```python
from build123d import *

# Parameters (mm, degrees)
EXTRUSION1_DEPTH = 18.3
ESQUISSE2_R      = 2
EXTRUSION2_DEPTH = 6.3


with BuildPart() as part:
    # Esquisse1 → Extrusion1 (new body)
    with BuildSketch(Plane.XY):
        with BuildLine():
            Line((0, 0), (30, 0))
            Line((30, 0), (30, 26.1))
            ThreePointArc((30, 26.1), (15, 41.1), (0, 26.1))
            Line((0, 26.1), (0, 0))
        make_face()
    extrude(amount=-EXTRUSION1_DEPTH)

    # Esquisse2 → Extrusion2 (cut)
    with BuildSketch(Plane.XY):
        with Locations((15, 26.6)):
            Circle(ESQUISSE2_R)
    extrude(amount=-EXTRUSION2_DEPTH, mode=Mode.SUBTRACT)


solid = part.part
```
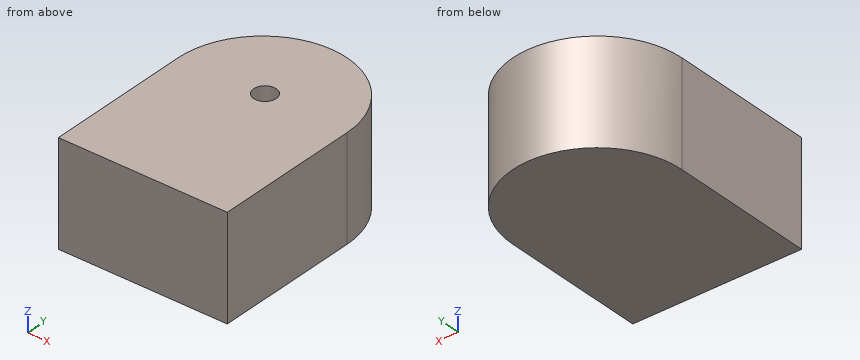
Geometry check sheet. Reference: the model listing, model coordinates, mm. Coordinates: 2 decimals unless noted, no trailing zeros. Order: outer loops, then holes, each group sorted by start corner. A loop starts at its lowest first (then second) coordinate and runs counter-clockwise, first axis right, second up.
Item 1: Scan lines: line 1 along Y through (x, z) = (15, -3.5); line 2 along Y through (x, z) = (16.5, -1); line 3 along Y through (x, z) = (15.5, -10.25). Record each from-to range of solid material in increasing order.
Item 2: Section check B-B (y = 26.6). Enter the section's corners in (x, z), plus the area to 3 significant figures.
Item 3: Section check C-C (z = -8.75). Enter the section's corners in (x, y), plus the area to 3 significant figures.
Item 4: Depth check by flat-ended pin: pin 1 (5 mm diameter, centred on x = 14.5, z = -12.5, fed in from +Y). Enter the tip coordinate at first touch or a pass-through.
Item 5: Section check D-D (y = 32.5). Enter the section's corners in (x, z).
Item 6: Section check A-A (x = 15). Enter the section's corners in (y, z).
Check sheet entries:
1. line 1: y = 0 to 24.6, 28.6 to 41.1
1. line 2: y = 0 to 25.28, 27.92 to 41.02
1. line 3: y = 0 to 41.09
2. outline: (0.01, -18.3) - (29.99, -18.3) - (29.99, 0) - (17, 0) - (17, -6.3) - (13, -6.3) - (13, 0) - (0.01, 0) - close
2. area: 523 mm2
3. outline: (0, 0) - (30, 0) - (30, 26.1) arc R15 ccw to (0, 26.1) - close
3. area: 1,140 mm2
4. pin 1: stops at y = 41.1
5. outline: (1.43, -18.3) - (28.57, -18.3) - (28.57, 0) - (1.43, 0) - close
6. outline: (0, -18.3) - (41.1, -18.3) - (41.1, 0) - (28.6, 0) - (28.6, -6.3) - (24.6, -6.3) - (24.6, 0) - (0, 0) - close
